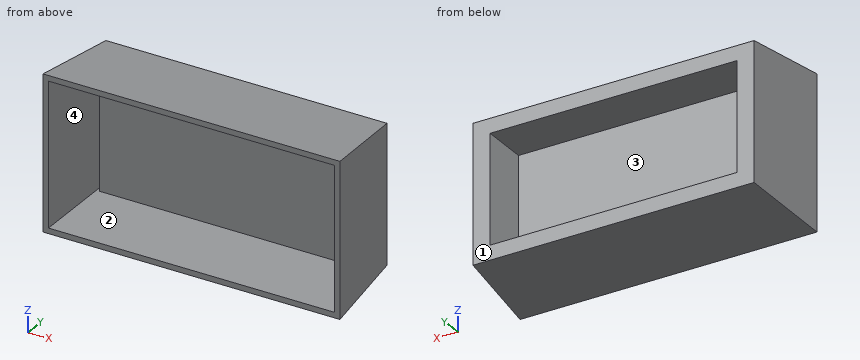
```python
from build123d import *

# Parameters (mm, degrees)
SKETCH1_W           = 164.136897748
SKETCH1_H           = 85.377660522
BOSS_EXTRUDE1_DEPTH = 50
BOSS_EXTRUDE1_TAPER = 5
SKETCH2_W           = 136.467789358
SKETCH2_H           = 60.390918278
CUT_EXTRUDE1_DEPTH  = 20
CUT_EXTRUDE1_TAPER  = 10
SHELL1_T            = -3


with BuildPart() as part:
    # Sketch1 → Boss-Extrude1 (new body)
    with BuildSketch(Plane(origin=(0, 0, 0), x_dir=(1, 0, 0), z_dir=(0, 1, 0))):
        Rectangle(SKETCH1_W, SKETCH1_H)
    extrude(amount=BOSS_EXTRUDE1_DEPTH, taper=BOSS_EXTRUDE1_TAPER)

    # Sketch2 → Cut-Extrude1 (cut)
    with BuildSketch(Plane(origin=(0, 50, 0), x_dir=(1, 0, 0), z_dir=(0, 1, 0))):
        Rectangle(SKETCH2_W, SKETCH2_H)
    extrude(amount=-CUT_EXTRUDE1_DEPTH, taper=CUT_EXTRUDE1_TAPER, mode=Mode.SUBTRACT)

    # Shell1
    shell1_openings = [part.faces().sort_by_distance(p)[0] for p in [
        (0, 0, 0),
    ]]
    offset(amount=SHELL1_T, openings=shell1_openings, kind=Kind.INTERSECTION)


solid = part.part
```
Work out the finished part from the listing and answer in its coordinate system (mm). Face numbers are marked on the shaded views. A direction names the side the tool comes from. Give positions to 0.01 mm unless a question says otherwise; leave off trailing zeros. Write item = value, one per line. Start each with the question number.
(1) Find the intervals of material crossed by probe 1 along Z at (x, y) = (59.5, 43); probe 2 along X at (y, z) = (38, 15); probe 3 along X at (y, z) = (33.5, 8), in increasing order. Write a range as from..to.
(2) Find section A-A on y = 32.5. Give the number of separate pieces and of enclosed holes in the cut face, and give its area (3 significant figures).
(3) Given pin 1 Ø4 at (x, y) = (-61, 8) entering from +Z; pin 2 Ø6 at (x, y) = (-26, 34.5) entering from +Z; pin 3 Ø4 at (y, z) = (43, 10.5) entering from -X, each flat-ended and moving along its own axis, determine where each tip first touches the part or whether it passes through.
(4) The mould has two halves that part along Z. Classify the marked faces 1 and 2: +Z half, -Z half, draft (parallel to the pull), parting line (faces both ways), or undercut.
(5) Which of the six approach directions +Z, -Z, +X, -X, +Y, -Y give full straight-line access (tool end or side, diameter ignored) to the marked faces 3 and 4?
From the geometry:
q1.probe_1 = -38.93..-35.92, -32.01..-28.96, 28.96..32.01, 35.92..38.93
q1.probe_2 = -78.74..-75.73, -69.16..-66.12, 66.12..69.16, 75.73..78.74
q1.probe_3 = -79.14..-76.13, -68.37..-65.32, 65.32..68.37, 76.13..79.14
q2.separate_pieces = 2
q2.enclosed_holes = 2
q2.area = 2,560 mm^2
q3.pin_1 = 42.16
q3.pin_2 = 39.93
q3.pin_3 = -78.48
q4.face_1 = draft
q4.face_2 = undercut
q5.face_3 = +Y
q5.face_4 = -Y
